Could you check a few things on this model? Use its own coordinates, in mm. Face numbers are marked on the shaded views. A direction names the side the tool comes from. Give positions to 0.01 mm unless a question says otherwise; leave off trailing zeros. Order: outer loops, then holes, each group sorted by start corner. A loop starts at its lowest first (then second) coordinate and runs counter-clockwise, first axis right, second up.
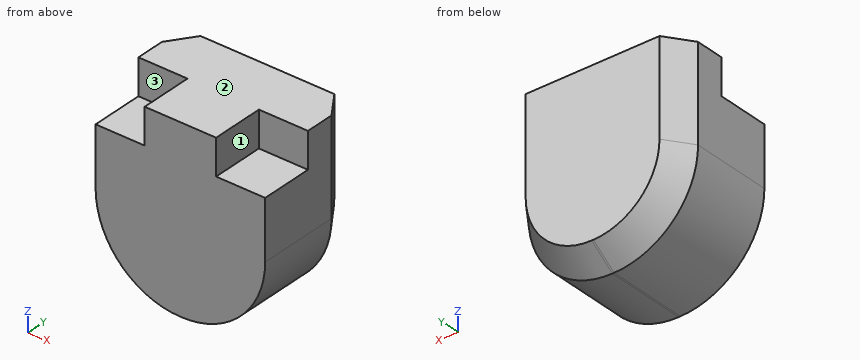
from build123d import *

# Parameters (mm, degrees)
F0_W     = 2.75
F0_H     = 2
F1_DEPTH = 6
F2_DEPTH = 2.95
F3_R     = 4.7
F4_SIZE2 = 1.4281480067
F4_SIZE  = 1


with BuildPart() as f1:
    # F0 (on Front) → F1 (new body)
    with BuildSketch(Plane.XZ):
        with Locations((3.375, 4)):
            Rectangle(F0_W, F0_H)
        Polygon((2, 3), (2, 5), (0, 5), (-2, 5), (-2, 3), align=None)
        Polygon((4.75, -5), (4.75, 3), (2, 3), (-2, 3), (-4.75, 3), (-4.75, -5), align=None)
        with Locations((-3.375, 4)):
            Rectangle(F0_W, F0_H)
    extrude(amount=-F1_DEPTH)

    # F0 (on Front) → F2 (cut)
    with BuildSketch(Plane.XZ):
        with Locations((-3.375, 4)):
            Rectangle(F0_W, F0_H)
        with Locations((3.375, 4)):
            Rectangle(F0_W, F0_H)
    extrude(amount=-F2_DEPTH, mode=Mode.SUBTRACT)

    # F3
    f3_edges = [f1.edges().sort_by_distance(p)[0] for p in [
        (-4.75, 3, -5),
        (4.75, 3, -5),
    ]]
    fillet(f3_edges, radius=F3_R)

    # F4
    f4_edges = [f1.edges().sort_by_distance(p)[0] for p in [
        (3.373402, 6, -3.623402),
        (-3.373402, 6, -3.623402),
        (0, 6, -5),
    ]]
    f4_side = f1.faces().sort_by_distance((0, 6, 0.437938))[0]
    chamfer(f4_edges, length=F4_SIZE, length2=F4_SIZE2, reference=f4_side)


solid = f1.part
Item 1: Imagine slicing it at C-C on y = 3.85. List the corners of the cut face in (x, z) for me.
Findings:
outline: (-4.75, -0.3) arc R4.7 ccw to (-0.05, -5) - (0.05, -5) arc R4.7 ccw to (4.75, -0.3) - (4.75, 5) - (-4.75, 5) - close
Item 2: Imagine slicing it at B-B on z = 2.5. List the corners of the cut face in (x, y) for me.
Findings:
outline: (-4.75, 0) - (4.75, 0) - (4.75, 4.57) - (3.75, 6) - (-3.75, 6) - (-4.75, 4.57) - close
Item 3: Imagine slicing it at D-D on z = 4. List the corners of the cut face in (x, y) for me.
Findings:
outline: (-4.75, 2.95) - (-2, 2.95) - (-2, 0) - (2, 0) - (2, 2.95) - (4.75, 2.95) - (4.75, 4.57) - (3.75, 6) - (-3.75, 6) - (-4.75, 4.57) - close
Item 4: For pin 1 (3 mm diameter, centred on y = 5.5, z = -3.5, fed in from -X); pin 2 (1.5 mm diameter, centred on x = 2, y = 3, fed in from -Z); pin 3 (2 mm diameter, centred on y = 1, z = 4.5, fed in from -X), each with a flat end and sliding along its axis, tell me the tip position at first contact or that it passes through.
Findings:
pin 1: stops at x = -4.29
pin 2: stops at z = -4.84
pin 3: stops at x = -2
Item 5: For the marked faces 1, 2 and 3, which set-ups out of +Z, -Z, +X, -X, +Y, -Y let a thin tool reach every point of the face, with its end or its side?
Findings:
face 1: +Z, +X, -Y
face 2: +Z, +X, -X, +Y, -Y
face 3: +Z, -X, -Y
Item 6: Imagine slicing it at A-A on y = 2.2. List the corners of the cut face in (x, z) for me, then the cut area to 3 significant figures.
Findings:
outline: (-4.75, -0.3) arc R4.7 ccw to (-0.05, -5) - (0.05, -5) arc R4.7 ccw to (4.75, -0.3) - (4.75, 3) - (2, 3) - (2, 5) - (-2, 5) - (-2, 3) - (-4.75, 3) - close
area: 74.5 mm2
Item 7: Please list where these lines run through material, in increasing order: line 1 along X through (y, z) = (2.1, 4.25); line 2 along Y through (x, z) = (3.5, 3.75); line 3 along Y through (x, z) = (4.25, -0.5).
Findings:
line 1: x = -2 to 2
line 2: y = 2.95 to 6
line 3: y = 0 to 5.28
